from build123d import *

# Parameters (mm, degrees)
F0_R     = 2.335
F1_DEPTH = 50.5726954
F2_R     = 5.08
F2_R_2   = 2.335
F3_DEPTH = 2.54
F4_R     = 0.889
F5_DEPTH = 12.7


with BuildPart() as f1:
    # F0 (on Top) → F1 (new body)
    with BuildSketch(Plane.XY):
        Circle(F0_R)
    extrude(amount=F1_DEPTH)

    # F2 (on face) → F3 (join)
    with BuildSketch(Plane(origin=(0, 0, 0), x_dir=(1, 0, 0), z_dir=(0, 0, -1))):
        Circle(F2_R)
        Circle(F2_R_2, mode=Mode.SUBTRACT)
        Circle(F2_R_2)
    extrude(amount=F3_DEPTH)

    # F4 (on Front) → F5 (cut, symmetric)
    with BuildSketch(Plane.XZ):
        with Locations((0, 48.1596954)):
            Circle(F4_R)
    extrude(amount=F5_DEPTH, both=True, mode=Mode.SUBTRACT)


solid = f1.part
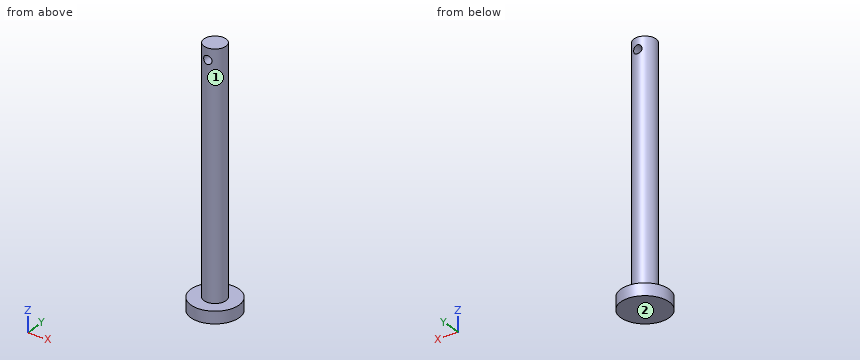
Design review of the part built by this model. Coordinates are the model's own, in mm. Face numbers are marked on the shaded views. A direction names the side the tool comes from. Round coordinates to 2 decimals unless told otherwise and drop trailing zeros. Loops run counter-clockwise (first coordinate to the right, second up) from the corner with the lowest first, then second, coordinate; pieces in that order, holes last. Notation, with made-up numbers: (8, 46.5) - (22, 46.5) arc R20 cw to (22, 84.5) - close; hole circle Ø9 at (83.25, -24.5). An arc over 180 degrees is marked (long way). One line per item, written item: value. Start each with the question number.
1) To check wall thickness, follow L1, parallel to Z at x = 0, y = -1.25; L2, parallel to Z at x = 2.5, y = -0.25; L3, parallel to Z at x = -0.75, y = -1. State the ranges of each line that lie inside material, in increasing order. Write a range as from..to.
2) For the marked faces 1 and 2, list the 3-axis set-ups (+Z, -Z, +X, -X, +Y, -Y) from which the entire face can be reached by the end or side of a thin tool; tool diameter is ignored.
3) Consider section A-A on x = 0. Give the boundary of the cut face in (y, z) (3 decimals).
4) Consider section C-C on z = 36. Give the boundary of the cut face in (x, y) (3 decimals).
5) Consider section D-D on x = -3.5. Give the boundary of the cut face in (y, z), then the cut area to 3 significant figures.
6) Insertion check: pin 1 Ø5 at (y, z) = (-1, 42.5) entering from -X (3 decimals); pin 2 Ø4 at (x, z) = (-1, 22.5) entering from -Y (3 decimals); pin 3 Ø4 at (x, z) = (3, 29.5) entering from -Y. Each pin has a flat end and moves straight along its axis. Give the tip position at first contact, or say it passes through.
7) Consider section B-B on y = 0. Give the boundary of the cut face in (x, z) (3 decimals), then the cut area to 3 significant figures.
Reported:
1. L1: z = -2.54..47.27, 49.05..50.57
1. L2: z = -2.54..0
1. L3: z = -2.54..47.68, 48.64..50.57
2. face 1: +Z
2. face 2: -Z, +X, -X, +Y, -Y
3. outline: (-5.08, -2.54) - (5.08, -2.54) - (5.08, 0) - (2.335, 0) - (2.335, 47.271) - (-2.335, 47.271) - (-2.335, 0) - (-5.08, 0) - close; (-2.335, 49.049) - (2.335, 49.049) - (2.335, 50.573) - (-2.335, 50.573) - close
4. outline: circle Ø4.67 at (0, 0)
5. outline: (-3.68, -2.54) - (3.68, -2.54) - (3.68, 0) - (-3.68, 0) - close
5. area: 18.7 mm^2
6. pin 1: stops at x = -2.335
6. pin 2: stops at y = -2.335
6. pin 3: stops at y = -2.11
7. outline: (-5.08, -2.54) - (5.08, -2.54) - (5.08, 0) - (2.335, 0) - (2.335, 50.573) - (-2.335, 50.573) - (-2.335, 0) - (-5.08, 0) - close; hole circle Ø1.778 at (0, 48.16)
7. area: 259 mm^2
